For this review, take the finished solid that the model builds, in its own axes (mm). Face numbers are marked on the shaded views. A direction names the side the tool comes from. Round coordinates to 2 decimals unless told otherwise and drop trailing zeros. Order: outer loops, then holes, each group sorted by start corner. A loop starts at its lowest first (then second) coordinate and runs counter-clockwise, first axis right, second up. Notation, with made-up numbers: M -3.5,4 L 46.5,4 A31 ccw 46.5,43 Z; hole C 18.25,6.5 d6. An arc over 180 degrees is marked long. Use a Markdown table: item, result.
from build123d import *

# Parameters (mm, degrees)
SKETCH1_W           = 19.5
SKETCH1_H           = 15
BOSS_EXTRUDE1_DEPTH = 8
CUT_EXTRUDE1_START  = -10
SKETCH3_R           = 3
CUT_EXTRUDE1_DEPTH  = 10


with BuildPart() as part:
    # Sketch1 → Revolve1 (revolve)
    with BuildSketch(Plane.XY, mode=Mode.PRIVATE) as revolve1_sk:
        with Locations((9.75, 7.5)):
            Rectangle(SKETCH1_W, SKETCH1_H)
    revolve(revolve1_sk.sketch.rotate(Axis((0, 0, 0), (1, 0, 0)), 90), axis=Axis((0, 0, 0), (1, 0, 0)))

    # Sketch2 → Boss-Extrude1 (add)
    with BuildSketch(Plane.ZY):
        with BuildLine():
            Line((-7, 0), (-7, 9.5))
            Line((-7, 9.5), (7, 9.5))
            Line((7, 9.5), (7, 0))
            ThreePointArc((7, 0), (0, -7), (-7, 0))
        make_face()
        with BuildLine():
            Line((-3, 0), (-3, 5.5))
            Line((-3, 5.5), (3, 5.5))
            Line((3, 5.5), (3, 0))
            ThreePointArc((3, 0), (0, -3), (-3, 0))
        make_face(mode=Mode.SUBTRACT)
    extrude(amount=BOSS_EXTRUDE1_DEPTH)

    # Sketch3 → Cut-Extrude1 (cut)
    with BuildSketch(Plane.ZY.offset(CUT_EXTRUDE1_START)):
        Circle(SKETCH3_R)
    extrude(amount=CUT_EXTRUDE1_DEPTH, mode=Mode.SUBTRACT)


solid = part.part
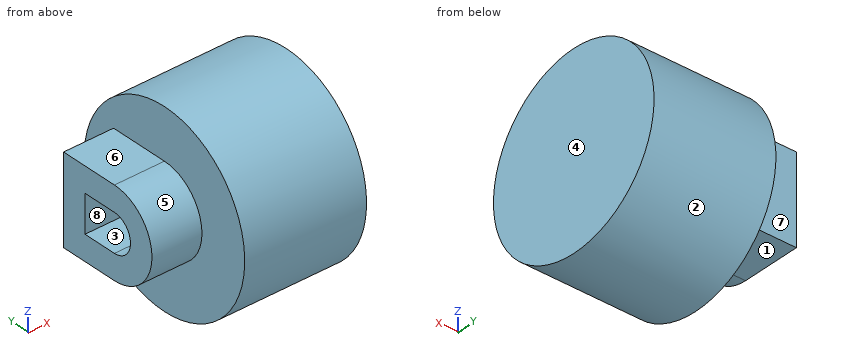
Q1. Add section B-B (z = 0). Write out the cut boundary in (x, y).
Determined:
| item | result |
|---|---|
| outline | M -8,-7 L 0,-7 L 0,-15 L 19.5,-15 L 19.5,15 L 0,15 L 0,9.5 L -8,9.5 L -8,5.5 L 0,5.5 L 0,3 L 10,3 L 10,-3 L -8,-3 Z |
Q2. Add section C-C (y = 8). Write out the cut boundary in (x, z), then the cut area to 3 significant figures.
Determined:
| item | result |
|---|---|
| outline | M -8,-7 L 0,-7 L 0,-12.69 L 19.5,-12.69 L 19.5,12.69 L 0,12.69 L 0,7 L -8,7 Z |
| area | 607 mm^2 |
Q3. Wall thickness on line 1 along Y through (x, z) = (6, 0); line 2 along Z through (x, y) = (-4.75, 8.5); line 3 along X through (y, z) = (-6.75, 4.5): over which ranges is each line inside the solid? List them lowest first. Write a range as [from, to].
Determined:
| item | result |
|---|---|
| line 1 | y = [-15, -3], [3, 15] |
| line 2 | z = [-7, 7] |
| line 3 | x = [0, 19.5] |
Q4. Draft analysis for pull direction Z (two halves, no side actions). For the marked faces 1, 2, 3 and 4, state which applies: pulls with the +Z half, pulls with the -Z half, needs draft (parallel to the pull), parting line crosses it, or undercut.
Determined:
| item | result |
|---|---|
| face 1 | pulls with the -Z half |
| face 2 | parting line crosses it |
| face 3 | undercut |
| face 4 | needs draft |
Q5. Machinability: for the marked faces 5, 6, 7 and 8, which of the approach directions +Z, -Z, +X, -X, +Y, -Y give a long, thin tool a straight path to every point of the face, cutting with its end or side? Answer none if there is none.
Determined:
| item | result |
|---|---|
| face 5 | -X, -Y |
| face 6 | +Z, -X, +Y, -Y |
| face 7 | +Z, -Z, -X, +Y |
| face 8 | -X |
Q6. Add section A-A (x = -3). Write out the cut boundary in (y, z), then the cut area to 3 significant figures.
Determined:
| item | result |
|---|---|
| outline | M 0,-7 L 9.5,-7 L 9.5,7 L 0,7 A7 ccw Z; hole M 0,-3 L 5.5,-3 L 5.5,3 L 0,3 A3 ccw Z |
| area | 163 mm^2 |
Q7. Clearance check with flat-ended pins moving along their axes: pin 1 (2.5 mm diameter, centred on x = -4.5, z = 2.5, fed in from +Y); pin 2 (5 mm diameter, centred on y = 8.5, z = -11.5, fed in from -X); pin 3 (12 mm diameter, centred on x = -3, y = -0.5, fed in from +Z); pin 4 (1 mm diameter, centred on x = 16.5, z = 7, fed in from +Y). State where each tip first meets the part, or that it passes through.
Determined:
| item | result |
|---|---|
| pin 1 | stops at y = 9.5 |
| pin 2 | stops at x = 0 |
| pin 3 | stops at z = 15 |
| pin 4 | stops at y = 13.52 |
Q8. Add section D-D (x = 17.75). Write out the cut boundary in (y, z).
Determined:
| item | result |
|---|---|
| outline | C 0,0 d30 |
